Build history of the part. All positions in model axes, mm. Round coordinates to 2 decimals unless told otherwise and drop trailing zeros. Loops run counter-clockwise (first coordinate to the right, second up) from the corner with the lowest first, then second, coordinate; pieces in that order, holes last.
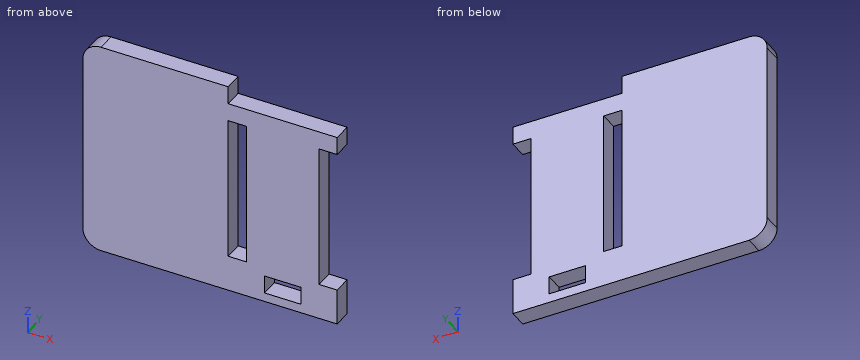
from build123d import *

# Parameters (mm, degrees)
BOSS_EXTRUDE1_DEPTH = 3.175
SKETCH2_W           = 6.35
SKETCH2_H           = 50.8
SKETCH2_W_2         = 12.7
SKETCH2_H_2         = 6.35
SKETCH2_W_3         = 38.1
CUT_EXTRUDE1_DEPTH  = 59.887477446


with BuildPart() as part:
    # Sketch1 → Boss-Extrude1 (new, symmetric)
    with BuildSketch(Plane(origin=(0, 0, 0), x_dir=(1, 0, 0), z_dir=(0, 1, 0))):
        with BuildLine():
            Line((44.45, -38.1), (-38.1, -38.1))
            ThreePointArc((-38.1, -38.1), (-42.590128061, -36.240128061), (-44.45, -31.75))
            Line((-44.45, -31.75), (-44.45, 31.75))
            ThreePointArc((-44.45, 31.75), (-42.590128061, 36.240128061), (-38.1, 38.1))
            Line((-38.1, 38.1), (44.45, 38.1))
            Line((44.45, 38.1), (44.45, -38.1))
        make_face()
    extrude(amount=BOSS_EXTRUDE1_DEPTH, both=True)

    # Sketch2 → Cut-Extrude1 (cut, through all)
    with BuildSketch(Plane.XZ.offset(3.175)):
        with Locations((9.525, 0)):
            Rectangle(SKETCH2_W, SKETCH2_H)
        with Locations((25.4, -31.75)):
            Rectangle(SKETCH2_W_2, SKETCH2_H_2)
        with Locations((41.275, 0)):
            Rectangle(SKETCH2_W, SKETCH2_H)
        with Locations((25.4, 34.925)):
            Rectangle(SKETCH2_W_3, SKETCH2_H_2)
    extrude(amount=-CUT_EXTRUDE1_DEPTH, mode=Mode.SUBTRACT)


solid = part.part
(1) Slice it at C-C on y = 0.5. List the corners of the cut face in (x, z) (3 decimals).
Responses:
outline: (-44.45, -31.75) arc R6.35 ccw to (-38.1, -38.1) - (44.45, -38.1) - (44.45, -25.4) - (38.1, -25.4) - (38.1, 25.4) - (44.45, 25.4) - (44.45, 31.75) - (6.35, 31.75) - (6.35, 38.1) - (-38.1, 38.1) arc R6.35 ccw to (-44.45, 31.75) - close; hole (6.35, -25.4) - (12.7, -25.4) - (12.7, 25.4) - (6.35, 25.4) - close; hole (19.05, -34.925) - (31.75, -34.925) - (31.75, -28.575) - (19.05, -28.575) - close
(2) Slice it at A-A on z = -16.5. List the corners of the cut face in (x, y) (3 decimals), plus the area to 3 significant figures.
Responses:
outline: (-44.45, -3.175) - (6.35, -3.175) - (6.35, 3.175) - (-44.45, 3.175) - close; (12.7, -3.175) - (38.1, -3.175) - (38.1, 3.175) - (12.7, 3.175) - close
area: 484 mm2
(3) Slice it at B-B on x = 20. List the corners of the cut face in (y, z) (3 decimals).
Responses:
outline: (-3.175, -38.1) - (3.175, -38.1) - (3.175, -34.925) - (-3.175, -34.925) - close; (-3.175, -28.575) - (3.175, -28.575) - (3.175, 31.75) - (-3.175, 31.75) - close
(4) Pin check, flat tip, straight feed: P1, Ø1.9, axis at x = 24, y = -0.5, coming from the +Z side. Stop position of the tip, or through.
Responses:
P1: stops at z = 31.75
(5) Probe line 1 (X direction, y = 2.5, z = -25); line 2 (X direction, y = -1, z = -29); line 3 (Z direction, x = 24.5, y = -0.75) (3 decimals). List the from-to ranges inside material, lowest first.
Responses:
line 1: x = -44.45 to 6.35, 12.7 to 38.1
line 2: x = -44.45 to 19.05, 31.75 to 44.45
line 3: z = -38.1 to -34.925, -28.575 to 31.75
